from build123d import *

# Parameters (mm, degrees)
SKETCH_1_W      = 15
SKETCH_1_H      = 15
EXTRUDE_1_DEPTH = 1
SKETCH_2_W      = 15
SKETCH_2_H      = 1
EXTRUDE_2_DEPTH = 15
M3X0_5_1_D      = 2.5
M3X0_5_2_D      = 2.5


with BuildPart() as part:
    # ｽｹｯﾁ1 → ﾎﾞｽ - 押し出し1 (new body)
    with BuildSketch(Plane.XY):
        with Locations((7.5, 7.5)):
            Rectangle(SKETCH_1_W, SKETCH_1_H)
    extrude(amount=EXTRUDE_1_DEPTH)

    # ｽｹｯﾁ2 → ﾎﾞｽ - 押し出し2 (add)
    with BuildSketch(Plane.XY.offset(1)):
        with Locations((7.5, 0.5)):
            Rectangle(SKETCH_2_W, SKETCH_2_H)
    extrude(amount=-EXTRUDE_2_DEPTH)

    # M3x0.5 ねじ穴1 (through all)
    with Locations(Plane.XY.offset(1)):
        with Locations((8, 8)):
            Hole(M3X0_5_1_D / 2)

    # M3x0.5 ねじ穴2 (through all)
    with Locations(Plane(origin=(0, 0, 0), x_dir=(-1, 0, 0), z_dir=(0, -1, 0))):
        with Locations((-8, 7)):
            Hole(M3X0_5_2_D / 2)


solid = part.part
Verification items for the finished model (mm, model axes). A direction names the side the tool comes from. Coordinates: 2 decimals unless noted, no trailing zeros. Loops run counter-clockwise (first coordinate to the right, second up) from the corner with the lowest first, then second, coordinate; pieces in that order, holes last. Notation, with made-up numbers: M 8.5,68 L 14.5,68 A18 ccw 14.5,83 Z; hole C 3,-28.5 d9. An arc over 180 degrees is marked long. One line per item, written item: value.
1. Gauge pin test, flat ends, axial feed: P1, Ø1.5, axis at x = 3.5, y = 9, coming from the -Z side; P2, Ø1.5, axis at x = 6, z = -1.5, coming from the +Y side. Record the tip position at first contact, or that the pin passes through.
Answers follow:
P1: z = 0
P2: y = 1
2. Section check D-D on x = 4.5. Record the cut outline in (y, z).
Answers follow:
outline: M 0,-14 L 1,-14 L 1,0 L 15,0 L 15,1 L 0,1 Z
3. Material ranges on line 1 along Z through (x, y) = (8, 0.7); line 2 along Y through (x, z) = (8, 0.7); line 3 along Y through (x, z) = (7, -0.75), recorded low to high. Write a range as from..to.
Answers follow:
line 1: -14..-8.25, -5.75..1
line 2: 0..6.75, 9.25..15
line 3: 0..1
4. Set-up check for faces 1 (the flat face through (7, 1, -5)), 2 (the flat face through (15, 0.8, -3.1)): record each of +Z, -Z, +X, -X, +Y, -Y from which the full face is reachable in a straight line by a thin tool's end or side.
Answers follow:
face 1: -Z, +X, -X, +Y
face 2: +Z, -Z, +X, +Y, -Y
5. Section check A-A on y = 8. Record the cut outline in (x, z).
Answers follow:
outline: M 0,0 L 6.75,0 L 6.75,1 L 0,1 Z; M 9.25,0 L 15,0 L 15,1 L 9.25,1 Z
6. Section check C-C on x = 8. Record the cut outline in (y, z), plus the area to 3 significant figures.
Answers follow:
outline: M 0,-14 L 1,-14 L 1,-8.25 L 0,-8.25 Z; M 0,-5.75 L 1,-5.75 L 1,0 L 6.75,0 L 6.75,1 L 0,1 Z; M 9.25,0 L 15,0 L 15,1 L 9.25,1 Z
area: 24.0 mm^2
7. Mould release check, pull along X, two halves, no side actions. Record for faces 3 (the flat face through (6, 8, 1)), 4 (the cylindrical face through (6.75, 0.51, -7.05)), 5 (the flat face through (0, 0.8, -3.1)): pulls with the +X half, pulls with the -X half, needs draft (parallel to the pull), parting line crosses it, or undercut.
Answers follow:
face 3: needs draft
face 4: undercut
face 5: pulls with the -X half
